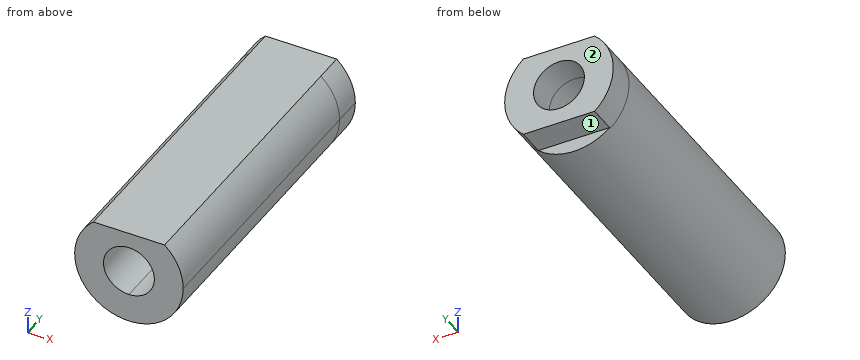
```python
from build123d import *

# Parameters (mm, degrees)
SKETCH_1_R             = 20.7
SKETCH_1_R_2           = 9.7
EXTRUDE_1_DEPTH        = 109.5
EXTRUDE_1_2_DEPTH      = 10
EXTRUDE_1_2_DEPTH_BACK = 1
SKETCH_2_W             = 45.579766756
SKETCH_2_H             = 31.21486686
SKETCH_3_R             = 9.7
CUT_EXTRUDE_1_DEPTH    = 124.886515749
SKETCH_4_W             = 48.064833826
SKETCH_4_H             = 7.030921468
CUT_EXTRUDE_2_DEPTH    = 114.745851724
SKETCH_5_R             = 31.7
SKETCH_5_R_2           = 20.7
CUT_EXTRUDE_1_2_DEPTH  = 124.886515749


with BuildPart() as part:
    # 草圖1 → Extrude 1 (new body)
    with BuildSketch(Plane(origin=(0, 0, 0), x_dir=(1, 0, 0), z_dir=(0, 1, 0))):
        Circle(SKETCH_1_R)
        Circle(SKETCH_1_R_2, mode=Mode.SUBTRACT)
    extrude(amount=EXTRUDE_1_DEPTH)

    # 草圖2 → Extrude 1 2 (add, two sides: drawn at the far end of the back side and taken through both)
    with BuildSketch(Plane(origin=(0, 110, 0), x_dir=(1, 0, 0), z_dir=(0, 1, 0)).offset(-EXTRUDE_1_2_DEPTH_BACK)):
        Rectangle(SKETCH_2_W, SKETCH_2_H)
    extrude(amount=EXTRUDE_1_2_DEPTH + EXTRUDE_1_2_DEPTH_BACK)

    # 草圖3 → Cut-Extrude 1 (cut, through all)
    with BuildSketch(Plane.XZ):
        with Locations(Location((0, 0, 0), (0, 0, 270))):
            Circle(SKETCH_3_R)
    extrude(amount=-CUT_EXTRUDE_1_DEPTH, mode=Mode.SUBTRACT)

    # 草圖4 → 除料-伸長2 (cut, through all)
    with BuildSketch(Plane(origin=(0, 109.5, 0), x_dir=(1, 0, 0), z_dir=(0, 1, 0))):
        with Locations((1.242533535, -19.122894164)):
            Rectangle(SKETCH_4_W, SKETCH_4_H)
    extrude(amount=-CUT_EXTRUDE_2_DEPTH, mode=Mode.SUBTRACT)

    # 草圖5 → Cut-Extrude 1 2 (cut, through all)
    with BuildSketch(Plane.XZ):
        Circle(SKETCH_5_R)
        Circle(SKETCH_5_R_2, mode=Mode.SUBTRACT)
    extrude(amount=-CUT_EXTRUDE_1_2_DEPTH, mode=Mode.SUBTRACT)


solid = part.part
```
The listing builds one solid part. Answer for the finished solid, in the listing's coordinates (mm). Face numbers are marked on the shaded views. A direction names the side the tool comes from. Coordinates: 2 decimals unless noted, no trailing zeros. Write each loop counter-clockwise with the first axis right and the second up, starting at its lowest first coordinate (ties: lowest second). Pieces come first, ordered by that corner, then holes. Notation, with made-up numbers: M 63,-2 L 75,-2 A15 ccw 75,4 Z; hole C 10.25,-13.75 d1. An arc over 180 degrees is marked long. Use a Markdown table: item, result. Add a question column.
1. Which of the six approach directions +Z, -Z, +X, -X, +Y, -Y give full straight-line access (tool end or side, diameter ignored) to the marked faces 1 and 2?
2. Section B-B (y = 83) is taken. Give the vertices of the cut face in (x, z), plus the area to 3 significant figures.
3. Straight lines are drawn through the part: line 1 along Z through (x, y) = (0, 59); line 2 along Z through (x, y) = (0, 116); line 3 along X through (y, z) = (111.5, 0). For each, find the intervals that lie inside material, in ascending order. Write a range as [from, to].
4. Section D-D (z = -14.5) is taken. Give the vertices of the cut face in (x, y).
5. Section A-A (x = 6) is taken. Give the vertices of the cut face in (y, z).
6. Section C-C (x = -2.5) is taken. Give the vertices of the cut face in (y, z).
7. Given P1, Ø1.5, axis at x = 5, y = 81.5, coming from the -Z side; P2, Ø5, axis at y = 45, z = -3, coming from the -X side; P3, Ø17.5, axis at x = 0, z = 0, coming from the +Y side; P4, Ø5, axis at x = -3, y = 114, coming from the -Z side, each flat-ended and moving along its own axis, determine where each tip first touches the part or whether it passes through.
Data:
| question | item | result |
|---|---|---|
| 1 | face 1 | -Z, +X, -X, +Y |
| 1 | face 2 | +Z, -Z, +X, -X, +Y |
| 2 | outline | M -13.6,15.61 A20.7 ccw long 13.6,15.61 Z; hole C 0,0 d19.4 |
| 2 | area | 956 mm2 |
| 3 | line 1 | z = [-20.7, -9.7], [9.7, 15.61] |
| 3 | line 2 | z = [-15.61, -9.7], [9.7, 15.61] |
| 3 | line 3 | x = [-20.7, -9.7], [9.7, 20.7] |
| 4 | outline | M -14.77,0 L 14.77,0 L 14.77,120 L -14.77,120 Z |
| 5 | outline | M 0,-19.81 L 109.5,-19.81 L 109.5,-15.61 L 120,-15.61 L 120,-7.62 L 0,-7.62 Z; M 0,7.62 L 120,7.62 L 120,15.61 L 0,15.61 Z |
| 6 | outline | M 0,-20.55 L 109.5,-20.55 L 109.5,-15.61 L 120,-15.61 L 120,-9.37 L 0,-9.37 Z; M 0,9.37 L 120,9.37 L 120,15.61 L 0,15.61 Z |
| 7 | P1 | stops at z = -20.26 |
| 7 | P2 | stops at x = -20.69 |
| 7 | P3 | passes through |
| 7 | P4 | stops at z = -15.61 |
